CAD build for the part. Positions are in the model's coordinates, mm. Face numbers are marked on the shaded views. A direction names the side the tool comes from. Round coordinates to 2 decimals unless told otherwise and drop trailing zeros. Write each loop counter-clockwise with the first axis right and the second up, starting at its lowest first coordinate (ties: lowest second). Pieces come first, ordered by that corner, then holes. Notation, with made-up numbers: M -19.5,-23.75 L 33.5,-23.75 A30 cw 33.5,-0.75 Z; hole C 48.25,38.25 d9. An arc over 180 degrees is marked long. Write each question's results on one line, items separated by ' | '. Start each with the question number.
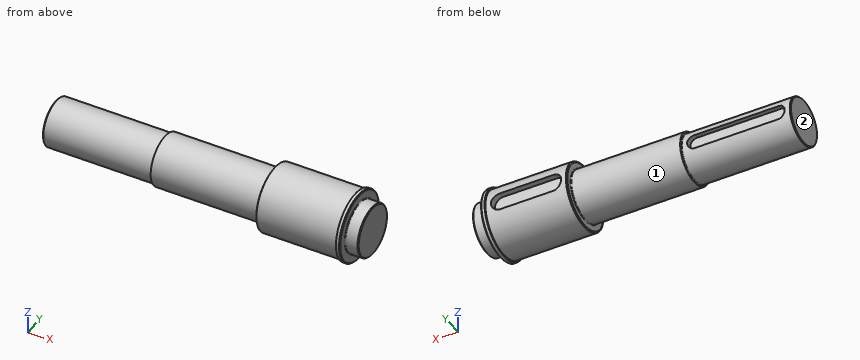
Autodesk Inventor part; units mm, degrees
ref_plane "Work Plane1" through (70.5, 30, 0) normal (0, 1, 0) x (-1, 0, 0)
ref_plane "Work Plane2" through (332, 42, 0) normal (0, 1, 0) x (-1, 0, 0)
ref_plane "YZ Plane" through (0, 0, 0) normal (1, 0, 0) x (0, 1, 0)
sketch "Sketch1" plane through (0, 0, 0) normal (0, 0, 1) x (1, 0, 0)
  point P0 (0, 0)
sketch "Sketch2" plane through (0, 0, 0) normal (0, 0, 1) x (1, 0, 0)
  line L0 (0, 0) -> (0, 29)
  line L1 (1, 30) -> (140, 30)
  line L2 (140, 30) -> (140, 32.5)
  line L3 (140, 32.5) -> (175, 32.5)
  line L4 (280, 37.5) -> (280, 42)
  line L5 (280, 42) -> (384, 42)
  line L6 (384, 42) -> (384, 44)
  line L7 (384, 44) -> (389, 44)
  line L8 (389, 44) -> (389, 39.5)
  line L9 (300, 32.5) -> (405, 32.5)
  line L10 (406, 31.5) -> (406, 0)
  line L11 (406, 0) -> (0, 0)
  line L12 (0, 29) -> (1, 30)
  line L13 (405, 32.5) -> (406, 31.5)
  line L14 (-81.2, 0) -> (487.2, 0)
  line L15 (389, 39.5) -> (389, 32.5)
  line L16 (389, 32.5) -> (300, 32.5)
  line L17 (280, 37.5) -> (280, 32.5)
  line L18 (280, 32.5) -> (175, 32.5)
  point P0 (0, 30)
  point P1 (406, 32.5)
  dimension "d0" = 30
  dimension "d1" = 140
  dimension "d2" = 32.5
  dimension "d3" = 140
  dimension "d4" = 104
  dimension "d5" = 5
  dimension "d6" = 17
  dimension "d7" = 32.5
  dimension "d8" = 42
  dimension "d9" = 2
  dimension "d10" = 1
  dimension "d11" = 45
  dimension "d12" = 1
  dimension "d13" = 45
revolve "Revolution1" add sketch "Sketch2" angle 360 about axis through (-10, 0, 0) along (1, 0, 0)
ref_plane "Work Plane1" through (70.5, 30, 0) normal (0, 1, 0) x (-1, 0, 0)
ref_plane "Work Plane2" through (332, 42, 0) normal (0, 1, 0) x (-1, 0, 0)
sketch "Sketch3" plane through (70.5, 30, 0) normal (0, 1, 0) x (-1, 0, 0)
  line L0 (54, 0) -> (-53, 0) construction
  line L1 (54, 9) -> (-53, 9)
  line L2 (-53, -9) -> (54, -9)
  arc A0 (54, -9) -> (54, 9) centre (54, 0) ccw
  arc A1 (-53, 9) -> (-53, -9) centre (-53, 0) ccw
  line L3 (-69.5, 32.5) -> (-69.5, -32.5)
  line L4 (0.5, -9) -> (0.5, 9) construction
  line L5 (70.5, 0) -> (-69.5, 0) construction
  line L6 (0.5, 0) -> (0.5, 9) construction
  line L7 (70.5, 29) -> (70.5, -29) construction
  point P0 (0.5, 0)
  dimension "d16" = 125
  dimension "d18" = 9
  dimension "d30" = 7.5
  dimension "d31" = 7.5
extrude "Extrusion1" cut sketch "Sketch3" against normal blind 7
sketch "Sketch4" plane through (332, 42, 0) normal (0, 1, 0) x (-1, 0, 0)
  line L0 (34, 0) -> (-34, 0) construction
  line L1 (34, -11) -> (-34, -11)
  line L2 (-34, 11) -> (34, 11)
  arc A0 (34, -11) -> (34, 11) centre (34, 0) ccw
  arc A1 (-34, 11) -> (-34, -11) centre (-34, 0) ccw
  line L3 (-52, 44) -> (-52, -44)
  line L4 (52, 42) -> (52, -42)
  line L5 (52, 42) -> (52, -42) construction
  line L6 (-52, 42) -> (-52, -42) construction
  line L7 (413.8, 0) -> (-155.3, 0) construction
  line L8 (-52, 0) -> (52, 0) construction
  line L9 (0, 11) -> (0, -11) construction
  line L10 (52, 42) -> (-52, 42) construction
  line L11 (0, 42) -> (0, -42) construction
  point P0 (332, 0)
  point P1 (0, 0)
  point P2 (0, 0)
  dimension "d22" = 11
  dimension "d32" = 90
extrude "Extrusion2" cut sketch "Sketch4" against normal blind 9
chamfer "Chamfer1" distance 1 angle 45 1 edges at (389, -44, 0) measured on face at (389, 1.3058, -39.927)
chamfer "Chamfer2" distance 1 angle 60 1 edges at (280, -42, 0) measured on face at (349.3333, 24.8095, 33.8893)
fillet "Fillet1" radius 1 1 edges at (280, -32.5, 0)
fillet "Fillet2" radius 1 1 edges at (140, -30, 0)
fillet "Fillet3" radius 1 1 edges at (389, -32.5, 0)
equation "\"d7\" = d2"
equation "\"d13\" = d11"
properties part number "GonjenoVratilo" material "Steel, Carbon"
1) 3-axis set-ups, long thin cutter, end or side, ignore diameter. For the marked faces 1 and 2: which of +Z, -Z, +X, -X, +Y, -Y reach the whole face in a straight line?
2) Drop flat-ended pins along their axis: pin 1 Ø1.7 at (x, y) = (57, 25) entering from -Z; pin 2 Ø4 at (x, y) = (326, 37.5) entering from -Z; pin 3 Ø1 at (x, z) = (112.5, -20) entering from -Y. Give the stop position or say it passes through.
3) Wall check: line 1 along X through (y, z) = (23.5, 29.5); line 2 along Z through (x, y) = (298, 37); line 3 along X through (y, z) = (24.5, -3). Give the ranges that are in metal, low to high. Write a range as from..to.
4) Saw through at A-A, the plane x = 224.5. Write the cut outline in (y, z).
Filled sheet:
1) face 1: -X | face 2: +Z, -Z, -X, +Y, -Y
2) pin 1: stops at z = -17.8 | pin 2: stops at z = -22.44 | pin 3: stops at y = -22.8
3) line 1: x = 280..389 | line 2: z = -19.87..-11, 11..19.87 | line 3: x = 0..8.01, 131.99..406
4) outline: C 0,0 d65
